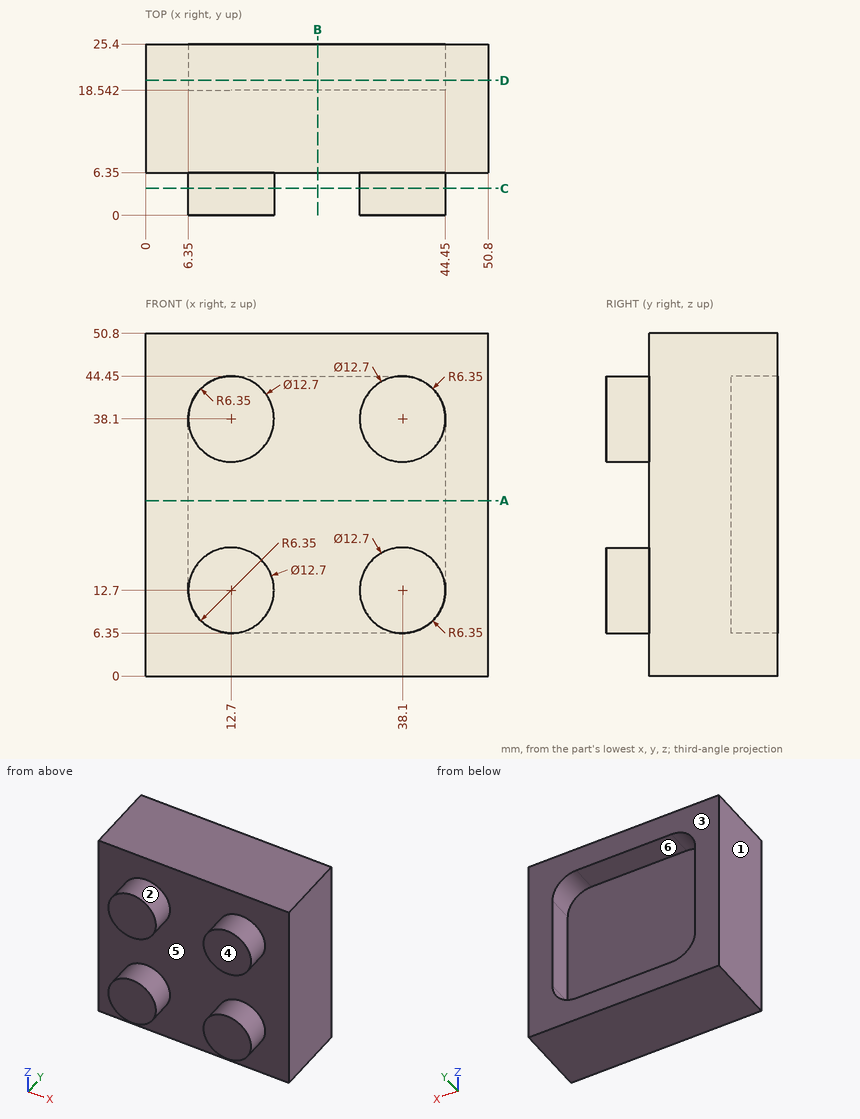
Could you check a few things on this drawing? It's one solid part, dimensions in mm from its lowest x, y, z. A direction names the side the tool comes from. Give positions to 0.01 mm unless a question says otherwise; leave off trailing zeros. Order: outer loops, then holes, each group sorted by start corner. A loop starts at its lowest first (then second) coordinate and runs counter-clockwise, first axis right, second up.
1. Suppose I cut it at A-A (z = 26). Write out the boundary of the cut face in (x, y).
Answers below:
outline: (0, 6.35) - (50.8, 6.35) - (50.8, 25.4) - (44.45, 25.4) - (44.45, 18.54) - (6.35, 18.54) - (6.35, 25.4) - (0, 25.4) - close
2. I need wall thicknesses on L1, parallel to X at y = 24, z = 26.5; L2, parallel to Y at x = 3.5, z = 30; L3, parallel to Y at x = 20, z = 21.5. Which ranges of each line are inside material? Lowest first, please.
Answers below:
L1: x = 0 to 6.35, 44.45 to 50.8
L2: y = 6.35 to 25.4
L3: y = 6.35 to 18.54
3. Which directions (+Z, -Z, +X, -X, +Y, -Y) give clear straight access to the entire face, cutting with the end or side of a thin tool? Please do the marked faces 4, 5 and 6.
Answers below:
face 4: +Z, -Z, +X, -X, -Y
face 5: -Y
face 6: +Y
4. For pin 1 (6 mm diameter, centred on x = 6, y = 3, fed in from +Z); pin 2 (11.5 mm diameter, centred on x = 33.5, z = 24.5, fed in from +Y); pin 3 (5 mm diameter, centred on x = 11.5, z = 28, fed in from -Y), each with a flat end and sliding along its axis, tell me the tip position at first contact or that it passes through.
Answers below:
pin 1: stops at z = 43.26
pin 2: stops at y = 18.54
pin 3: stops at y = 6.35
5. Suppose I cut it at B-B (x = 25.5). Write out the boundary of the cut face in (y, z), plus the area to 3 significant figures.
Answers below:
outline: (6.35, 0) - (25.4, 0) - (25.4, 6.35) - (18.54, 6.35) - (18.54, 44.45) - (25.4, 44.45) - (25.4, 50.8) - (6.35, 50.8) - close
area: 706 mm2
6. Suppose I cut it at D-D (y = 20). Write out the boundary of the cut face in (x, z), plus the area to 3 significant figures.
Answers below:
outline: (0, 0) - (50.8, 0) - (50.8, 50.8) - (0, 50.8) - close; hole (6.35, 12.7) arc R6.35 ccw to (12.7, 6.35) - (38.1, 6.35) arc R6.35 ccw to (44.45, 12.7) - (44.45, 38.1) arc R6.35 ccw to (38.1, 44.45) - (12.7, 44.45) arc R6.35 ccw to (6.35, 38.1) - close
area: 1,160 mm2
7. Thinking about a two-plate mould opening in X: for the marked faces 1, 2 and 3, which applies, +X half, -X half, draft (parallel to the pull), parting line (faces both ways), or undercut?
Answers below:
face 1: -X half
face 2: undercut
face 3: draft
8. Suppose I cut it at C-C (y = 4). Write out the boundary of the cut face in (x, z), plus the area to 3 significant figures.
Answers below:
outline: circle Ø12.7 at (12.7, 12.7); circle Ø12.7 at (12.7, 38.1); circle Ø12.7 at (38.1, 12.7); circle Ø12.7 at (38.1, 38.1)
area: 507 mm2
